Here's how the part is built. I have some questions about the finished solid (model axes, mm). A direction names the side the tool comes from. Coordinates: 2 decimals unless noted, no trailing zeros. Order: outer loops, then holes, each group sorted by start corner. A loop starts at its lowest first (then second) coordinate and runs counter-clockwise, first axis right, second up.
```python
from build123d import *

# Parameters (mm, degrees)
SKETCH1_R                = 14
BOSS_EXTRUDE1_DEPTH      = 9.25
SKETCH2_R                = 12.5
BOSS_EXTRUDE2_DEPTH      = 0.5
BOSS_EXTRUDE3_START      = 0.5
SKETCH3_R                = 12.5
BOSS_EXTRUDE3_DEPTH      = 0.5
SKETCH4_R                = 14
BOSS_EXTRUDE4_DEPTH      = 5
BOSS_EXTRUDE5_START      = 1
SKETCH5_R                = 14
BOSS_EXTRUDE5_DEPTH      = 1
BOSS_EXTRUDE6_START      = 4
SKETCH6_R                = 4
BOSS_EXTRUDE6_DEPTH      = 4
BOSS_EXTRUDE7_START      = 11
SKETCH7_R                = 4
BOSS_EXTRUDE7_DEPTH      = 11
FILLET4_SIZE             = 2
BOSS_EXTRUDE8_DEPTH      = 3
SKETCH10_R               = 4.5
SKETCH9_R                = 2.5
FILLET5_R                = 3
CUT_EXTRUDE1_START       = -2
CUT_EXTRUDE1_DEPTH       = 2
BOSS_EXTRUDE9_DEPTH      = 8
BOSS_EXTRUDE9_DEPTH_BACK = 17
SKETCH16_R               = 0.675
BOSS_EXTRUDE10_DEPTH     = 9
SKETCH18_R               = 0.5
CUT_EXTRUDE2_DEPTH       = 9
SCALE1_SCALE             = 2
SKETCH19_R               = 19.428126758
CUT_EXTRUDE3_DEPTH       = 35


with BuildPart() as part:
    # Sketch1 → Boss-Extrude1 (new, symmetric)
    with BuildSketch(Plane(origin=(0, 0, 0), x_dir=(1, 0, 0), z_dir=(0, 1, 0))):
        with Locations(Location((0, 0, 0), (0, 0, 270))):
            Circle(SKETCH1_R)
    extrude(amount=BOSS_EXTRUDE1_DEPTH, both=True)

    # Sketch2 → Boss-Extrude2 (add)
    with BuildSketch(Plane(origin=(0, 9.25, 0), x_dir=(1, 0, 0), z_dir=(0, 1, 0))):
        with Locations(Location((0, 0, 0), (0, 0, 270))):
            Circle(SKETCH2_R)
    extrude(amount=BOSS_EXTRUDE2_DEPTH)

    # Sketch3 → Boss-Extrude3 (add)
    with BuildSketch(Plane.XZ.offset(9.25).offset(BOSS_EXTRUDE3_START)):
        with Locations(Location((0, 0, 0), (0, 0, 90))):
            Circle(SKETCH3_R)
    extrude(amount=-BOSS_EXTRUDE3_DEPTH)

    # Sketch4 → Boss-Extrude4 (add)
    with BuildSketch(Plane.XZ.offset(9.75)):
        with Locations(Location((0, 0, 0), (0, 0, 90))):
            Circle(SKETCH4_R)
    extrude(amount=BOSS_EXTRUDE4_DEPTH)

    # Sketch5 → Boss-Extrude5 (add)
    with BuildSketch(Plane(origin=(0, 9.75, 0), x_dir=(1, 0, 0), z_dir=(0, 1, 0)).offset(BOSS_EXTRUDE5_START)):
        with Locations(Location((0, 0, 0), (0, 0, 270))):
            Circle(SKETCH5_R)
    extrude(amount=-BOSS_EXTRUDE5_DEPTH)

    # Sketch6 → Boss-Extrude6 (add)
    with BuildSketch(Plane(origin=(0, 10.75, 0), x_dir=(1, 0, 0), z_dir=(0, 1, 0)).offset(BOSS_EXTRUDE6_START)):
        with BuildLine():
            ThreePointArc((6.560632788, 3.783884599), (3.142489225, 4.325265354), (1.571341079, 7.408817209))
            Line((1.571341079, 7.408817209), (2.245059227, 13.818817209))
            ThreePointArc((2.245059227, 13.818817209), (0, 14), (-2.245059227, 13.818817209))
            Line((-2.245059227, 13.818817209), (-1.571341079, 7.408817209))
            ThreePointArc((-1.571341079, 7.408817209), (-3.019559024, 4.156066449), (-6.560632788, 3.783884599))
            Line((-6.560632788, 3.783884599), (-12.4487147, 6.405427568))
            ThreePointArc((-12.4487147, 6.405427568), (-13.314791228, 4.326237921), (-13.836237609, 2.135071152))
            Line((-13.836237609, 2.135071152), (-7.531774982, 0.795016253))
            ThreePointArc((-7.531774982, 0.795016253), (-4.885749132, -1.587476124), (-5.62603513, -5.070247918))
            Line((-5.62603513, -5.070247918), (-9.938788028, -9.86004526))
            ThreePointArc((-9.938788028, -9.86004526), (-8.228993532, -11.326237921), (-6.306205891, -12.499270669))
            Line((-6.306205891, -12.499270669), (-3.083551855, -6.917470143))
            ThreePointArc((-3.083551855, -6.917470143), (0, -5.13718065), (3.083551855, -6.917470143))
            Line((3.083551855, -6.917470143), (6.306205891, -12.499270669))
            ThreePointArc((6.306205891, -12.499270669), (8.228993532, -11.326237921), (9.938788028, -9.86004526))
            Line((9.938788028, -9.86004526), (5.62603513, -5.070247918))
            ThreePointArc((5.62603513, -5.070247918), (5.084654375, -1.652104355), (7.531774982, 0.795016253))
            Line((7.531774982, 0.795016253), (13.836237609, 2.135071152))
            ThreePointArc((13.836237609, 2.135071152), (13.314791228, 4.326237921), (12.4487147, 6.405427568))
            Line((12.4487147, 6.405427568), (6.560632788, 3.783884599))
        make_face()
        with Locations(Location((0, 0, 0), (0, 0, 270))):
            Circle(SKETCH6_R, mode=Mode.SUBTRACT)
    extrude(amount=-BOSS_EXTRUDE6_DEPTH)

    # Sketch7 → Boss-Extrude7 (add)
    with BuildSketch(Plane(origin=(0, 10.75, 0), x_dir=(1, 0, 0), z_dir=(0, 1, 0)).offset(BOSS_EXTRUDE7_START)):
        with Locations(Location((0, 0, 0), (0, 0, 270))):
            Circle(SKETCH7_R)
    extrude(amount=-BOSS_EXTRUDE7_DEPTH)

    # Fillet4
    fillet4_edges = [part.edges().sort_by_distance(p)[0] for p in [
        (0, 14.75, -14),
        (-13.314791228, 14.75, -4.326237921),
        (-8.228993532, 14.75, 11.326237921),
        (8.228993532, 14.75, 11.326237921),
        (13.314791228, 14.75, -4.326237921),
    ]]
    chamfer(fillet4_edges, length=FILLET4_SIZE)

    # Sketch8 → Boss-Extrude8 (add)
    with BuildSketch(Plane(origin=(0, 21.75, 0), x_dir=(1, 0, 0), z_dir=(0, 1, 0))):
        Polygon((-2.862387208, 5), (2.862387208, 5), (6.179011998, 0), (2.862387208, -5), (-2.862387208, -5), (-6.179011998, 0), align=None)
    extrude(amount=BOSS_EXTRUDE8_DEPTH)

    # Sketch10 → Loft1 section 0
    with BuildSketch(Plane(origin=(0, 24.75, 0), x_dir=(1, 0, 0), z_dir=(0, 1, 0))):
        Circle(SKETCH10_R)
    # Sketch9 → Loft1 section 1
    with BuildSketch(Plane(origin=(0, 34, 0), x_dir=(1, 0, 0), z_dir=(0, 1, 0))):
        Circle(SKETCH9_R)
    loft()

    # Fillet5
    fillet5_edges = [part.edges().sort_by_distance(p)[0] for p in [
        (-2.5, 34, 0),
    ]]
    fillet(fillet5_edges, radius=FILLET5_R)

    # Sketch12 → Cut-Extrude1 (cut)
    with BuildSketch(Plane.XZ.offset(14.75).offset(CUT_EXTRUDE1_START)):
        with BuildLine():
            ThreePointArc((3, 13.674794331), (0, 14), (-3, 13.674794331))
            Line((-3, 13.674794331), (-3, 8))
            ThreePointArc((-3, 8), (0, 5), (3, 8))
            Line((3, 8), (3, 13.674794331))
        make_face()
        with BuildLine():
            Line((-8, 3), (-13.674794331, 3))
            ThreePointArc((-13.674794331, 3), (-14, 0), (-13.674794331, -3))
            Line((-13.674794331, -3), (-8, -3))
            ThreePointArc((-8, -3), (-5, 0), (-8, 3))
        make_face()
        with BuildLine():
            Line((12.289759461, 6.705356992), (6.260800415, 2.483834421))
            ThreePointArc((6.260800415, 2.483834421), (4.967798056, 0), (6.260800415, -2.483834421))
            Line((6.260800415, -2.483834421), (12.289759461, -6.705356992))
            ThreePointArc((12.289759461, -6.705356992), (14, 0), (12.289759461, 6.705356992))
        make_face()
        with BuildLine():
            Line((-3, -8), (-3, -13.674794331))
            ThreePointArc((-3, -13.674794331), (0, -14), (3, -13.674794331))
            Line((3, -13.674794331), (3, -8))
            ThreePointArc((3, -8), (0, -5), (-3, -8))
        make_face()
    extrude(amount=CUT_EXTRUDE1_DEPTH, mode=Mode.SUBTRACT)

    # Sketch14 → Boss-Extrude9 (add, two sides: drawn at the far end of the back side and taken through both)
    with BuildSketch(Plane(origin=(14, 0, 0), x_dir=(0, 0, -1), z_dir=(1, 0, 0)).offset(-BOSS_EXTRUDE9_DEPTH_BACK)):
        with BuildLine():
            Line((-3, -13), (3, -13))
            ThreePointArc((3, -13), (3.75, -13.75), (3, -14.5))
            Line((3, -14.5), (-3, -14.5))
            ThreePointArc((-3, -14.5), (-3.75, -13.75), (-3, -13))
        make_face()
    extrude(amount=BOSS_EXTRUDE9_DEPTH + BOSS_EXTRUDE9_DEPTH_BACK)

    # Sketch16 → Boss-Extrude10 (add)
    with BuildSketch(Plane(origin=(22, 0, 0), x_dir=(0, 0, -1), z_dir=(1, 0, 0))):
        with Locations((-2.25, -13.75)):
            Circle(SKETCH16_R)
        with Locations((0, -13.75)):
            Circle(SKETCH16_R)
        with Locations((2.25, -13.75)):
            Circle(SKETCH16_R)
    extrude(amount=BOSS_EXTRUDE10_DEPTH)

    # Sketch18 → Cut-Extrude2 (cut)
    with BuildSketch(Plane(origin=(31, 0, 0), x_dir=(0, 0, -1), z_dir=(1, 0, 0))):
        with Locations((-2.25, -13.75)):
            Circle(SKETCH18_R)
        with Locations((2.25, -13.75)):
            Circle(SKETCH18_R)
        with Locations((0, -13.75)):
            Circle(SKETCH18_R)
    extrude(amount=-CUT_EXTRUDE2_DEPTH, mode=Mode.SUBTRACT)


with BuildPart() as part_1:
    # Scale1: scaled about (0.135762453, 0.409238593, -0.000649103)
    add(part.part.scale(SCALE1_SCALE).moved(Location((-0.135762453, -0.409238593, 0.000649103))))

    # Sketch19 → Cut-Extrude3 (cut)
    with BuildSketch(Plane.XZ.offset(18.90923893)):
        with Locations(Location((0, 0, 0), (0, 0, 270))):
            Circle(SKETCH19_R)
    extrude(amount=-CUT_EXTRUDE3_DEPTH, mode=Mode.SUBTRACT)


solid = part_1.part
```
Q1. We'd pull the mould along Y, two halves only. Please class faces 6 (the cylindrical face through (9.8, -29.7, 0.1)), 7 (the cylindrical face through (6.23, 25.15, -8.59)), 8 (the conical face through (24.64, 27.06, -7.98)): pulls with the +Y half, pulls with the -Y half, needs draft (parallel to the pull), parting line crosses it, or undercut.
Q2. For faces 1 (the flat face through (-6.136, -28, 22)), 2 (the flat face through (27, -26.409, 0)), 3 (the flat face through (-21.592, 25.147, -2.948)), 4 (the flat face through (8.952, 46.049, 4.931)), 5 (the flat face through (-22, -28, 6.001)), which set-ups out of +Z, -Z, +X, -X, +Y, -Y let a thin tool reach every point of the face, with its end or its side?
Q3. If we section it at A-A on x = 32: Write out the boundary of the cut face in (y, z).
Q4. If we section it at C-C on y = 39: Write out the boundary of the cut face in (x, z).
Q5. Will these pins go through, and if not, where does the flat tip stop? pin 1 (10 mm diameter, centred on y = -8.5, z = -7, fed in from -X); pin 2 (4 mm diameter, centred on x = 19, z = -20, fed in from +Y); pin 3 (5 mm diameter, centred on x = -3, z = -15, fed in from -Y).
Q6. I need wall thicknesses on L1, parallel to Y at x = -21, z = 16; L2, parallel to Y at x = -13, z = 9; L3, parallel to X at y = -16, z = 25. Which ranges of each line are inside material? Lowest first, please.
Q7. If we section it at B-B on y = -9.5: Write out the boundary of the cut face in (x, z), then the cut area to 3 significant figures.
Reply:
1. face 6: needs draft
1. face 7: undercut
1. face 8: pulls with the +Y half
2. face 1: +Z, -Y
2. face 2: +X
2. face 3: -X, +Y
2. face 4: +Z, +X, +Y
2. face 5: -X, -Y
3. outline: (-29.41, -6) arc R1.5 ccw to (-26.41, -6) - (-26.41, 6) arc R1.5 ccw to (-29.41, 6) - close
4. outline: circle Ø16 at (-0.14, 0)
5. pin 1: stops at x = -28.06
5. pin 2: stops at y = 21.09
5. pin 3: stops at y = -25.91
6. L1: y = -29.91 to -19.91, -18.91 to 18.09, 19.09 to 21.09
6. L2: y = -29.91 to -18.91, 16.09 to 21.09
6. L3: x = -12.75 to 12.48
7. outline: circle Ø56 at (-0.14, 0); hole circle Ø38.86 at (0, 0)
7. area: 1,280 mm2
